Source: CAD feature listing. Evaluate the final solid. Frame: model axes, mm. Round coordinates to 2 decimals unless told otherwise and drop trailing zeros. Write each loop counter-clockwise with the first axis right and the second up, starting at its lowest first coordinate (ties: lowest second). Pieces come first, ordered by that corner, then holes. Notation, with made-up numbers: M 75,8 L 102,8 A35 ccw 102,47 Z; hole C 62.25,-40 d4. An arc over 180 degrees is marked long. Answer in a Markdown table with one row per item. Add a question column.
Item 1: Contact query for flat-ended pins moving along their axis: pin 1 (3 mm diameter, centred on x = -148.5, z = 268, fed in from -Y); pin 2 (4 mm diameter, centred on y = -77.5, z = 428, fed in from +X). Output: stop coordinate, or through.
Item 2: Material intervals for probe 1 along X at (y, z) = (-48, 771); probe 2 along X at (y, z) = (-186, 858.5); probe 3 along Y at (x, z) = (29, 358.5), sorted ascending.
Item 3: Cut plane C-C on y = -72. Return loops of the section in (x, z), and give its area (3 significant figures).
Item 4: Cut plane A-A on y = -149. Return loops of the section in (x, z).
Item 5: Cut plane D-D on x = -276. Return loops of the section in (y, z), and give its area (3 significant figures).
Item 6: Cut plane B-B on z = 684. Return loops of the section in (x, y), and give its area (3 significant figures).
Item 7: Mould query, pull axis X, two halves, no side actions, for faces 1 (the face through (-758.072, -123.42, 493)), 2 (the face through (-761.06, -123.17, 493)), 3 (the face through (760.786, -119.897, 493)). Classes: released by +X, released by -X, zero draft, split by the parting line, or undercut.
Autodesk Inventor part; units mm, degrees
ref_plane "YZ Plane" through (0, 0, 0) normal (1, 0, 0) x (0, 1, 0)
ref_plane "XZ Plane" through (0, 0, 0) normal (0, 1, 0) x (-1, 0, 0)
ref_plane "XY Plane" through (0, 0, 0) normal (0, 0, 1) x (1, 0, 0)
sketch "Sketch1" plane through (0, 0, 0) normal (0, 0, 1) x (1, 0, 0)
  line L0 (-750, 0) -> (750, 0) construction
  line L1 (750, 0) -> (750, -2700) construction
  line L2 (750, -2700) -> (-750, -2700) construction
  line L3 (-750, -2700) -> (-750, 0) construction
  line L4 (800, 50) -> (-800, 50) construction
  line L5 (-800, 50) -> (-800, -2750) construction
  line L6 (-800, -2750) -> (800, -2750) construction
  line L7 (800, -2750) -> (800, 50) construction
  line L8 (-850, 100) -> (850, 100) construction
  line L9 (850, 100) -> (850, -2800) construction
  line L10 (850, -2800) -> (-850, -2800) construction
  line L11 (-850, -2800) -> (-850, 100) construction
  arc A0 (750, 0) -> (745.2706, 0.6314) centre (0, -5600) ccw construction
  line L12 (-750, -2100) -> (750, -2100) construction
  line L13 (114.1118, -2698.3696) -> (750, -2100) construction
  arc A1 (750, -2100) -> (770.156, -238.4205) centre (-10250, -1050) ccw construction
  line L14 (750, 0) -> (749.6018, -2.9735) construction
  arc A2 (750, -3.0268) -> (0, 47) centre (-0.2, -5603) ccw construction
  line L15 (750, 0) -> (747.0136, -0.2851) construction
  arc A3 (767.1641, -238.6409) -> (747.4657, -5.0326) centre (-10252.9895, -1050.2527) ccw construction
  arc A4 (750.4522, -4.7486) -> (745.2706, 0.6314) centre (744.4791, -5.3162) ccw
  arc A5 (747.4657, -5.0326) -> (744.8748, -2.3426) centre (744.4792, -5.3164) ccw construction
  line L16 (750, -2100) -> (752.9864, -2100.2851) construction
  arc A6 (752.9864, -2100.2851) -> (771.2831, -213.263) centre (-10246.9891, -1050.0292) ccw construction
  line L17 (750, -2100) -> (752.0559, -2102.1848) construction
  line L18 (752.0559, -2102.1848) -> (752.0559, -2102.1848) construction
  arc A7 (749.1768, -2100.7746) -> (750.1074, -2098.8746) centre (747.1209, -2098.5898) ccw construction
  line L19 (0, -2697) -> (110, -2697) construction
  line L20 (112.0559, -2696.1848) -> (685.3133, -2156.7506) construction
  arc A8 (110, -2700) -> (114.1118, -2698.3696) centre (110, -2694) ccw construction
  arc A9 (110, -2697) -> (112.0559, -2696.1848) centre (110, -2694) ccw construction
  line L21 (685.3133, -2156.7506) -> (687.3692, -2158.9354) construction
  line L22 (752.0559, -2102.1848) -> (671.2185, -2178.2526) construction
  line L23 (671.2185, -2178.2526) -> (669.1626, -2176.0678) construction
  arc A10 (747.4657, -5.0326) -> (747.0136, -0.2851) centre (-10252.9895, -1050.2527) ccw construction
  arc A11 (745.2706, 0.6314) -> (0, 50) centre (0, -5600) ccw
  arc A12 (750.4522, -4.7486) -> (750, 0) centre (-10250, -1050) ccw construction
  line L24 (770.156, -238.4205) -> (767.1641, -238.6409) construction
  line L25 (768.2917, -213.4901) -> (771.2831, -213.263) construction
  arc A13 (770.156, -238.4205) -> (750.4522, -4.7486) centre (-10250, -1050) ccw
  line L26 (0, 100) -> (0, 50) construction
  line L27 (0, -2700) -> (0, -2697) construction
  line L28 (0, 47) -> (0, 0) construction
  line L29 (0, 50) -> (0, 47) construction
  arc A14 (752.0559, -2102.1848) -> (752.9864, -2100.2851) centre (749.9998, -2099.9999) ccw construction
  point P0 (0, -2750)
  dimension "d54" = 1500
  dimension "d55" = 2700
  dimension "d58" = 2100
  dimension "d68" = 6
  dimension "d70" = 3
  dimension "d75" = 3
  dimension "d83" = 6
  dimension "d86" = 3
  dimension "d112" = 239.271
  dimension "d113" = 50
  dimension "d114" = 50
  dimension "d115" = 3
  dimension "d117" = 110
  dimension "d118" = 25
  dimension "d119" = 111
  dimension "d120" = 25
contour flange "Contour Flange2" sketch "Sketch1" thickness 3 bend radius 3 width 1000 along (0, 0, 1) mid plane no both sides no wall seen from (760.924, -121.5323, 0) lies toward (-0.9964637, -0.0840242, 0) curves A13 A4 A11
bend "Bend2"
corner "Corner2"
mirror "Mirror2" about plane through (0, 0, 0) normal (1, 0, 0)
equation "\"d36\" = Thickness"
equation "\"d37\" = BendReliefWidth"
equation "\"d38\" = BendReliefDepth"
equation "\"d39\" = MinimumRemnant"
equation "\"d40\" = TransitionRadius"
equation "\"d42\" = BendRadius"
equation "\"d44\" = CornerReliefSize"
equation "\"d45\" = GapSize"
equation "\"d46\" = JacobiRadiusSize"
equation "\"BendRadius\" = Thickness"
equation "\"BendReliefWidth\" = Thickness"
equation "\"BendReliefDepth\" = 0.5 * Thickness"
equation "\"CornerReliefSize\" = 4 * Thickness"
equation "\"MinimumRemnant\" = 2 * Thickness"
equation "\"TransitionRadius\" = BendRadius"
equation "\"JacobiRadiusSize\" = BendRadius"
equation "\"GapSize\" = Thickness"
properties part number "МОО 033 лист спина базовый" material "Stainless Steel AISI 304"
Results below:
| question | item | result |
|---|---|---|
| 1 | pin 1 | y = 45.01 |
| 1 | pin 2 | x = 757.3 |
| 2 | probe 1 | -754.48 to -751.46, 751.46 to 754.48 |
| 2 | probe 2 | -766.17 to -763.16, 763.16 to 766.17 |
| 2 | probe 3 | 46.93 to 49.93 |
| 3 | outline | M -756.64,0 L -753.62,0 L -753.62,1000 L -756.64,1000 Z; M 753.62,0 L 756.64,0 L 756.64,1000 L 753.62,1000 Z |
| 3 | area | 6,020 mm2 |
| 4 | outline | M -763.21,0 L -760.2,0 L -760.2,1000 L -763.21,1000 Z; M 760.2,0 L 763.21,0 L 763.21,1000 L 760.2,1000 Z |
| 5 | outline | M 40.25,0 L 43.25,0 L 43.25,1000 L 40.25,1000 Z |
| 5 | area | 3,000 mm2 |
| 6 | outline | M -770.16,-238.42 L -767.16,-238.64 A11046.82 cw -747.47,-5.03 A3 cw -744.87,-2.34 A5646.99 cw 0,47 A5646.99 cw 744.87,-2.34 A3 cw 747.47,-5.03 A11046.82 cw 767.16,-238.64 L 770.16,-238.42 A11049.82 ccw 750.45,-4.75 A6 ccw 745.27,0.63 A5649.99 ccw 0,50 A5649.99 ccw -745.27,0.63 A6 ccw -750.45,-4.75 A11049.82 ccw Z |
| 6 | area | 5,930 mm2 |
| 7 | face 1 | undercut |
| 7 | face 2 | released by -X |
| 7 | face 3 | released by +X |
